from build123d import *

# Parameters (mm, degrees)
F_02_KEYWAY_DEPTH = 2.5


with BuildPart() as part:
    # 草图1 → 旋转1 (revolve)
    with BuildSketch(Plane.XY, mode=Mode.PRIVATE) as revolve_1_sk:
        Polygon((0, 0), (0, 7), (0.5, 7.5), (18, 7.5), (18, 9), (50, 9), (50, 12.5), (58.5, 12.5), (58.5, 15.5), (65.5, 15.5), (65.5, 12.5), (89.5, 12.5), (89.5, 9), (105, 9), (105.5, 8.5), (105.5, 0), align=None)
    revolve(revolve_1_sk.sketch.rotate(Axis((-5, 0, 0), (1, 0, 0)), 90), axis=Axis((-5, 0, 0), (1, 0, 0)))

    # 草图2 → 02_KEYWAY (cut)
    with BuildSketch(Plane(origin=(0, 9, 0), x_dir=(1, 0, 0), z_dir=(0, 1, 0))):
        with BuildLine():
            Line((28, 1.5), (38, 1.5))
            ThreePointArc((38, 1.5), (39.5, 0), (38, -1.5))
            Line((38, -1.5), (28, -1.5))
            ThreePointArc((28, -1.5), (26.5, 0), (28, 1.5))
        make_face()
    extrude(amount=-F_02_KEYWAY_DEPTH, mode=Mode.SUBTRACT)


solid = part.part
Here's how the part is built. I have some questions about the finished solid (model axes, mm). A direction names the side the tool comes from. Round coordinates to 2 decimals unless told otherwise and drop trailing zeros. Write each loop counter-clockwise with the first axis right and the second up, starting at its lowest first coordinate (ties: lowest second). Pieces come first, ordered by that corner, then holes.
1. Suppose I cut it at B-B (y = 0). List the corners of the cut face in (x, z) for me, and give its area (3 significant figures).
2. I need wall thicknesses on L1, parallel to X at y = -8, z = -1; L2, parallel to X at y = 11, z = -3; L3, parallel to Z at x = 95, y = 3. Which ranges of each line are inside material? Lowest first, please.
3. Suppose I cut it at C-C (x = 87). List the corners of the cut face in (y, z) for me.
4. Suppose I cut it at D-D (x = 15). List the corners of the cut face in (y, z) for me, and give its area (3 significant figures).
5. If we mould it in two halves opening along Z, with no side actions, what happens to faces 4 (the cylindrical face through (34.224, -6.083, -6.633)), 5 (the cylindrical face through (26.5, 7.8, 0)), 6 (the flat face through (105.5, 0, 0))? For each: released by +Z, released by -Z, zero draft, split by the parting line, or undercut.
6. For faces 1 (the flat face through (33, 8, 1.5)), 2 (the cylindrical face through (97.358, -6.083, -6.633)), 3 (the cylindrical face through (9.372, -6.324, 4.032)), which set-ups out of +Z, -Z, +X, -X, +Y, -Y let a thin tool reach every point of the face, with its end or its side?
7. Will these pins go through, and if not, where does the flat tip stop? pin 1 Ø10 at (x, z) = (63, 2.5) entering from +Y; pin 2 Ø0.7 at (x, y) = (31.5, 8) entering from -Z; pin 3 Ø2 at (x, y) = (43.5, 2) entering from -Z; pin 4 Ø0.7 at (x, y) = (32, 8) entering from +Z.
Answer sheet:
1. outline: (0, -7) - (0.5, -7.5) - (18, -7.5) - (18, -9) - (50, -9) - (50, -12.5) - (58.5, -12.5) - (58.5, -15.5) - (65.5, -15.5) - (65.5, -12.5) - (89.5, -12.5) - (89.5, -9) - (105, -9) - (105.5, -8.5) - (105.5, 8.5) - (105, 9) - (89.5, 9) - (89.5, 12.5) - (65.5, 12.5) - (65.5, 15.5) - (58.5, 15.5) - (58.5, 12.5) - (50, 12.5) - (50, 9) - (18, 9) - (18, 7.5) - (0.5, 7.5) - (0, 7) - close
1. area: 2,160 mm2
2. L1: x = 18 to 105.5
2. L2: x = 50 to 89.5
2. L3: z = -8.49 to 8.49
3. outline: circle Ø25 at (0, 0)
4. outline: circle Ø15 at (0, 0)
4. area: 177 mm2
5. face 4: split by the parting line
5. face 5: undercut
5. face 6: zero draft
6. face 1: +Y
6. face 2: +X
6. face 3: -X
7. pin 1: stops at y = 15.5
7. pin 2: stops at z = -4.74
7. pin 3: stops at z = -8.94
7. pin 4: stops at z = 4.74
